from build123d import *

# Parameters (mm, degrees)
CONG_1_R         = 1
CONG_2_R         = 1
COQUE3_OUTLINE_R = 30.5
COQUE3_DEPTH     = 19


# Read off the part's stored shape, not the designer's step: Coque3
with BuildPart() as part:
    # Esquisse1 → Révolution1 (revolve)
    with BuildSketch(Plane.XY, mode=Mode.PRIVATE) as r_volution1_sk:
        Polygon((0, 0), (32.5, 0), (32.5, 15), (31.5, 15), (31.5, 20), (0, 20), align=None)
    revolve(r_volution1_sk.sketch.rotate(Axis((0, 0, 0), (0, -1, 0)), 90), axis=Axis((0, 0, 0), (0, -1, 0)))

    # Congé1
    cong_1_edges = [part.edges().sort_by_distance(p)[0] for p in [
        (0, 20, -31.5),
    ]]
    fillet(cong_1_edges, radius=CONG_1_R)

    # Congé2
    cong_2_edges = [part.edges().sort_by_distance(p)[0] for p in [
        (0, 15, -32.5),
    ]]
    fillet(cong_2_edges, radius=CONG_2_R - 0.0001)  # a hair under: the kernel refuses the full size

    # Coque3 outline → Coque3 (cut)
    with BuildSketch(Plane(origin=(0, 0, 0), x_dir=(1, 0, 0), z_dir=(0, 1, 0))):
        Circle(COQUE3_OUTLINE_R)
    extrude(amount=COQUE3_DEPTH, mode=Mode.SUBTRACT)


solid = part.part
Part model, mm, in its own coordinate system. A direction names the side the tool comes from. Round coordinates to 2 decimals unless told otherwise and drop trailing zeros. Loops run counter-clockwise (first coordinate to the right, second up) from the corner with the lowest first, then second, coordinate; pieces in that order, holes last. Notation, with made-up numbers: (68.5, 67.25) - (101.5, 67.25) arc R22 cw to (101.5, 81.25) - close; hole circle Ø9 at (19, -19). An arc over 180 degrees is marked (long way). Answer as a JSON object with one key per item and string values.
Item 1: Pull direction X, two halves, no side cores. Call faces 1 (the face through (-29, 0, 10)), 2 (the face through (-9.76, 7.1, 31)), 3 (the face through (-24.204, 9.367, 18.559)), 4 (the face through (0, 19, 0)): pulls with the +X half, pulls with the -X half, needs draft (parallel to the pull), parting line crosses it, or undercut.
Output:
{"face 1": "needs draft", "face 2": "parting line crosses it", "face 3": "undercut", "face 4": "undercut"}
Item 2: Band-saw the part on D-D on y = 4.5. List the corners of the cut face in (x, z).
Output:
{"outline": "circle Ø65 at (0, 0); hole circle Ø61 at (0, 0)"}
Item 3: Band-saw the part on C-C on y = 16.75. List the corners of the cut face in (x, z).
Output:
{"outline": "circle Ø63 at (0, 0); hole circle Ø61 at (0, 0)"}
Item 4: Pin check, flat tips, straight feed: pin 1 (18.5 mm diameter, centred on x = 9, z = 8, fed in from -Y); pin 2 (3 mm diameter, centred on y = 9.5, z = 25, fed in from -X); pin 3 (5 mm diameter, centred on y = 7.5, z = -11, fed in from +X). Stop position of each tip, or through.
Output:
{"pin 1": "y = 19", "pin 2": "x = -22.45", "pin 3": "x = 31.37"}
Item 5: Tool access for faces 5 (the face through (0, 20, 0)), 6 (the face through (-31.232, 17.028, -4.101)): list every direction of +Z, -Z, +X, -X, +Y, -Y with a clear straight run to the whole face (end or side of a thin tool).
Output:
{"face 5": "+Z, -Z, +X, -X, +Y", "face 6": "+Y"}
Item 6: Wall check: L1, parallel to X at y = 7.75, z = 0; L2, parallel to Y at x = -15, z = 6; L3, parallel to Z at x = -10, y = 18. Give the ranges that are in metal, low to high.
Output:
{"L1": "-32.5 to -30.5, 30.5 to 32.5", "L2": "19 to 20", "L3": "-29.87 to -28.81, 28.81 to 29.87"}
